```python
from build123d import *

# Parameters (mm, degrees)
F0_R     = 35
F1_DEPTH = 3
F2_R     = 1.55
F3_DEPTH = 3.001
F4_R     = 7
F5_DEPTH = 10
F6_R     = 4
F7_DEPTH = 13.001


with BuildPart() as f1:
    # F0 (on Top) → F1 (new body)
    with BuildSketch(Plane.XY):
        Circle(F0_R)
    extrude(amount=F1_DEPTH)

    # F2 (on face) → F3 (cut, through all)
    with BuildSketch(Plane.XY.offset(3)):
        with Locations((0, 30)):
            Circle(F2_R)
        with Locations((-25.980762, 15)):
            Circle(F2_R)
        with Locations((-25.980762, -15)):
            Circle(F2_R)
        with Locations((25.980762, 15)):
            Circle(F2_R)
        with Locations((25.980762, -15)):
            Circle(F2_R)
        with Locations((0, -30)):
            Circle(F2_R)
    extrude(amount=-F3_DEPTH, mode=Mode.SUBTRACT)

    # F4 (on face) → F5 (join)
    with BuildSketch(Plane.XY.offset(3)):
        Circle(F4_R)
    extrude(amount=F5_DEPTH)

    # F6 (on face) → F7 (cut, through all)
    with BuildSketch(Plane.XY.offset(13)):
        Circle(F6_R)
    extrude(amount=-F7_DEPTH, mode=Mode.SUBTRACT)


solid = f1.part
```
Design review of the part built by this model. Coordinates are the model's own, in mm. Coordinates: 2 decimals unless noted, no trailing zeros. Write each loop counter-clockwise with the first axis right and the second up, starting at its lowest first coordinate (ties: lowest second). Pieces come first, ordered by that corner, then holes.
1) Add section A-A (y = 0). Write out the cut boundary in (x, z), plus the area to 3 significant figures.
2) Add section D-D (y = 15). Write out the cut boundary in (x, z).
3) Insertion check: pin 1 (5 mm diameter, centred on x = -17.5, z = 2, fed in from +Y); pin 2 (3.5 mm diameter, centred on x = 25.98, y = -15, fed in from +Z). Each pin has a flat end and moves straight along its axis. Give the tip position at first contact, or say it passes through.
4) Mouldability with a two-part tool opening along Y and no side actions: class faces 1 (the cylindrical face through (-0.867, -3.905, 6.591)), 2 (the flat face through (7, 0, 0)), 3 (the cylindrical face through (6.466, -2.681, 7.93)) as +Y half, -Y half, draft (parallel to the pull), parting line (faces both ways), or undercut.
5) To check wall thickness, follow L1, parallel to Y at x = 0, z = 1.85; L2, parallel to Y at x = 0, z = 9.5; L3, parallel to Z at x = -6.5, y = -11. State the ranges of each line that lie inside material, in increasing order.
6) Add section C-C (z = 1). Write out the cut boundary in (x, y).
7) Add section B-B (x = 0). Write out the cut boundary in (y, z).
Check result:
1. outline: (-35, 0) - (-4, 0) - (-4, 13) - (-7, 13) - (-7, 3) - (-35, 3) - close; (4, 0) - (35, 0) - (35, 3) - (7, 3) - (7, 13) - (4, 13) - close
1. area: 246 mm2
2. outline: (-31.62, 0) - (-27.53, 0) - (-27.53, 3) - (-31.62, 3) - close; (-24.43, 0) - (24.43, 0) - (24.43, 3) - (-24.43, 3) - close; (27.53, 0) - (31.62, 0) - (31.62, 3) - (27.53, 3) - close
3. pin 1: stops at y = 31.62
3. pin 2: stops at z = 3
4. face 1: undercut
4. face 2: draft
4. face 3: parting line
5. L1: y = -35 to -31.55, -28.45 to -4, 4 to 28.45, 31.55 to 35
5. L2: y = -7 to -4, 4 to 7
5. L3: z = 0 to 3
6. outline: circle Ø70 at (0, 0); hole circle Ø3.1 at (-25.98, -15); hole circle Ø3.1 at (-25.98, 15); hole circle Ø8 at (0, 0); hole circle Ø3.1 at (0, -30); hole circle Ø3.1 at (0, 30); hole circle Ø3.1 at (25.98, -15); hole circle Ø3.1 at (25.98, 15)
7. outline: (-35, 0) - (-31.55, 0) - (-31.55, 3) - (-35, 3) - close; (-28.45, 0) - (-4, 0) - (-4, 13) - (-7, 13) - (-7, 3) - (-28.45, 3) - close; (4, 0) - (28.45, 0) - (28.45, 3) - (7, 3) - (7, 13) - (4, 13) - close; (31.55, 0) - (35, 0) - (35, 3) - (31.55, 3) - close
